Study the drawing (mm; zero at the part's minimum x, y, z) and answer. Give positions to 0.01 mm unless a question says otherwise; leave off trailing zeros. Order: outer loops, then holes, each group sorted by start corner. A loop starts at its lowest first (then second) coordinate and runs counter-clockwise, first axis right, second up.
Item 1: A cutting plane is placed at C-C (z = 9.75). State how many separate pieces and enclosed holes the cut face has, plus the area to 3 significant figures.
Item 2: Find the intervals of material crossed by line 1 along Y through (x, z) = (19.05, 4) (1 decimal); line 2 along X through (y, z) = (129.5, 4.5); line 3 along Y through (x, z) = (125.5, 7.75), in increasing order.
Item 3: A cutting plane is placed at D-D (x = 158). Write down the section's boundary in (y, z), plus the area to 3 significant figures.
Item 4: Given pin 1 Ø4 at (x, y) = (209.55, 41.275) entering from +Z; pin 2 Ø1 at (x, z) = (156, 4.5) entering from +Y; pin 3 Ø4 at (x, z) = (119.5, 5.5) entering from -Y, each flat-ended and moving along its own axis, determine where each tip first touches the part or whether it passes through.
Item 5: A cutting plane is placed at B-B (y = 221). Write down the section's boundary in (x, z).
Item 6: A cutting plane is placed at A-A (x = 209.55). Write down the section's boundary in (y, z) (1 decimal).
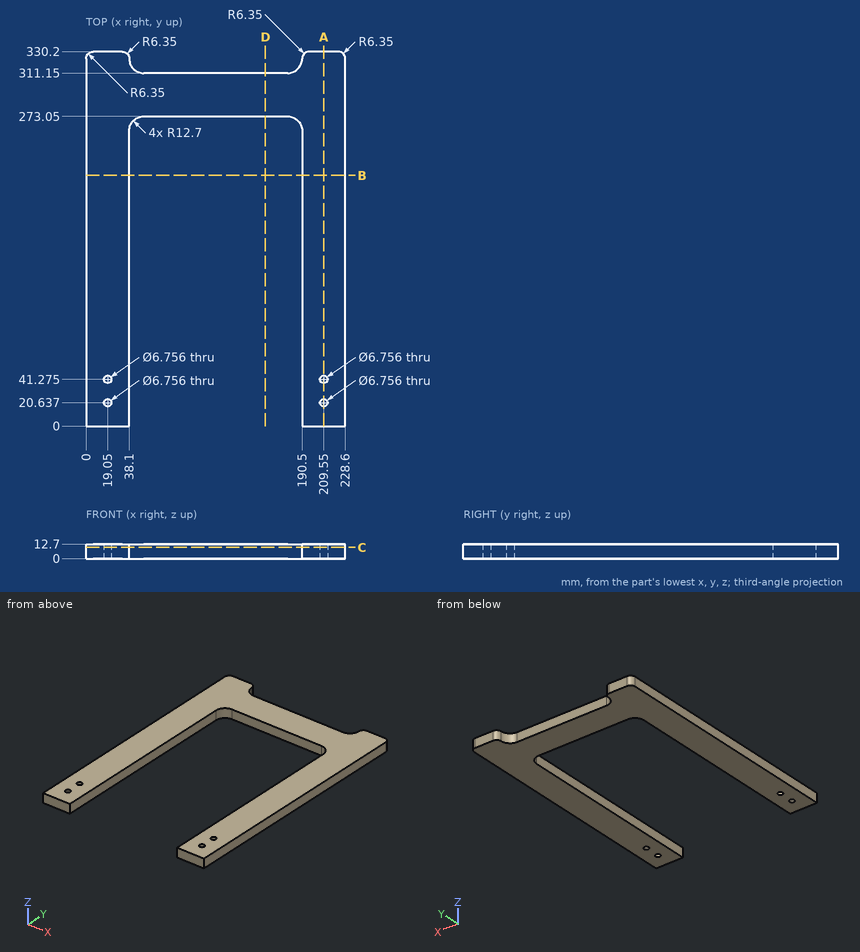
Response values:
1. separate pieces: 1
1. enclosed holes: 4
1. area: 30,900 mm2
2. line 1: y = 0 to 17.3, 24 to 37.9, 44.7 to 330.2
2. line 2: x = 0 to 38.1, 190.5 to 228.6
2. line 3: y = 273.05 to 311.15
3. outline: (273.05, 0) - (311.15, 0) - (311.15, 12.7) - (273.05, 12.7) - close
3. area: 484 mm2
4. pin 1: passes through
4. pin 2: stops at y = 311.15
4. pin 3: stops at y = 273.05
5. outline: (0, 0) - (38.1, 0) - (38.1, 12.7) - (0, 12.7) - close; (190.5, 0) - (228.6, 0) - (228.6, 12.7) - (190.5, 12.7) - close
6. outline: (0, 0) - (17.3, 0) - (17.3, 12.7) - (0, 12.7) - close; (24, 0) - (37.9, 0) - (37.9, 12.7) - (24, 12.7) - close; (44.7, 0) - (330.2, 0) - (330.2, 12.7) - (44.7, 12.7) - close
